from build123d import *

# Parameters (mm, degrees)
F0_W     = 47
F0_H     = 114
F1_DEPTH = 1
F0_W_2   = 36
F0_H_2   = 32.15
F2_DEPTH = 3
F3_R     = 3
F4_W     = 8
F4_H     = 32.15
F5_DEPTH = 2
F4_W_2   = 1.6
F4_H_2   = 10
F6_DEPTH = 2


with BuildPart() as f1:
    # F0 (on Top) → F1 (new body)
    with BuildSketch(Plane.XY):
        Rectangle(F0_W, F0_H)
        Polygon((18, 23.75), (20.25, 23.75), (20.25, -53.75), (-20.25, -53.75), (-20.25, 23.75), (-18, 23.75), (-18, 55.9), (18, 55.9), align=None, mode=Mode.SUBTRACT)
    extrude(amount=F1_DEPTH)

    # F0 (on Top) → F2 (join)
    with BuildSketch(Plane.XY):
        Polygon((20.25, -53.75), (20.25, 23.75), (18, 23.75), (-18, 23.75), (-20.25, 23.75), (-20.25, -53.75), align=None)
        with Locations((0, 39.825)):
            Rectangle(F0_W_2, F0_H_2)
    extrude(amount=F2_DEPTH)

    # F3
    f3_edges = [f1.edges().sort_by_distance(p)[0] for p in [
        (23.5, -57, 0.5),
        (-23.5, -57, 0.5),
        (23.5, 57, 0.5),
        (-23.5, 57, 0.5),
    ]]
    fillet(f3_edges, radius=F3_R)

    # F4 (on face) → F5 (cut)
    with BuildSketch(Plane.XY.offset(3)):
        Polygon((-10, -53.75), (10, -53.75), (10, 23.75), (4, 23.75), (-4, 23.75), (-10, 23.75), align=None)
        with Locations((0, 39.825)):
            Rectangle(F4_W, F4_H)
    extrude(amount=-F5_DEPTH, mode=Mode.SUBTRACT)

    # F4 (on face) → F6 (join)
    with BuildSketch(Plane.XY.offset(3)):
        with Locations((-10.3, 39.825)):
            Rectangle(F4_W_2, F4_H_2)
        with Locations((10.3, 39.825)):
            Rectangle(F4_W_2, F4_H_2)
    extrude(amount=F6_DEPTH)


solid = f1.part
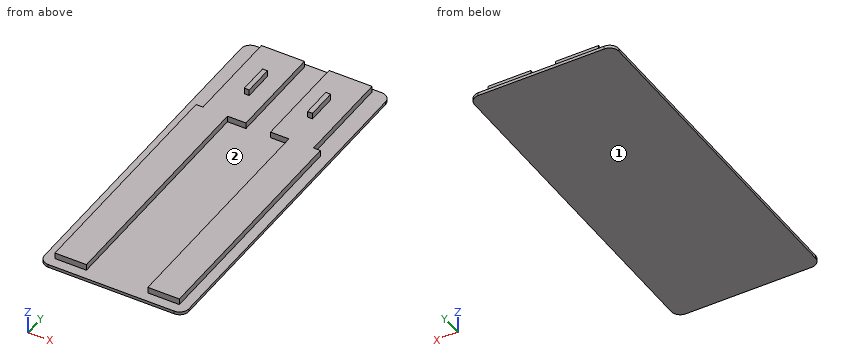
Can you work these out from the model? Positions are in its coordinate system, mm. Face numbers are marked on the shaded views. Give positions to 0.01 mm unless a question says otherwise; leave off trailing zeros. Loops run counter-clockwise (first coordinate to the right, second up) from the corner with the lowest first, then second, coordinate; pieces in that order, holes last. Notation, with made-up numbers: M 62,-18 L 80,-18 A11 ccw 80,2 Z; hole C 40.5,-18 d4. An arc over 180 degrees is marked long. One line per item, written item: value.
1) Imagine slicing it at C-C on x = 6. Write out the boundary of the cut face in (y, z).
Geometry check:
outline: M -57,0 L 57,0 L 57,1 L 55.9,1 L 55.9,3 L 23.75,3 L 23.75,1 L -57,1 Z
2) Imagine slicing it at B-B on x = 15. Write out the boundary of the cut face in (y, z).
Geometry check:
outline: M -57,0 L 57,0 L 57,1 L 55.9,1 L 55.9,3 L -53.75,3 L -53.75,1 L -57,1 Z
3) I'm going to push flat-ended pins straight in: pin 1 (1 mm diameter, centred on y = 46.5, z = 2, fed in from -X); pin 2 (1.6 mm diameter, centred on y = -33, z = 2, fed in from +X); pin 3 (2 mm diameter, centred on x = 19.5, z = 2.5, fed in from +Y). Where does each tip first touch, or does it pass through?
Geometry check:
pin 1: stops at x = -18
pin 2: stops at x = 20.25
pin 3: stops at y = 23.75
4) Please list where these lines run through material, in increasing order: line 1 (X direction, y = 41.5, z = 3.15); line 2 (X direction, y = 52, z = 2.8); line 3 (Y direction, x = 18.5, z = 2.9).
Geometry check:
line 1: x = -11.1 to -9.5, 9.5 to 11.1
line 2: x = -18 to -4, 4 to 18
line 3: y = -53.75 to 23.75
5) Thinking about a two-plate mould opening in X: for the marked faces 1 and 2, which applies, +X half, -X half, draft (parallel to the pull), parting line (faces both ways), or undercut?
Geometry check:
face 1: draft
face 2: undercut
6) Imagine slicing it at A-A on y = -16. Write out the boundary of the cut face in (x, z).
Geometry check:
outline: M -23.5,0 L 23.5,0 L 23.5,1 L 20.25,1 L 20.25,3 L 10,3 L 10,1 L -10,1 L -10,3 L -20.25,3 L -20.25,1 L -23.5,1 Z
